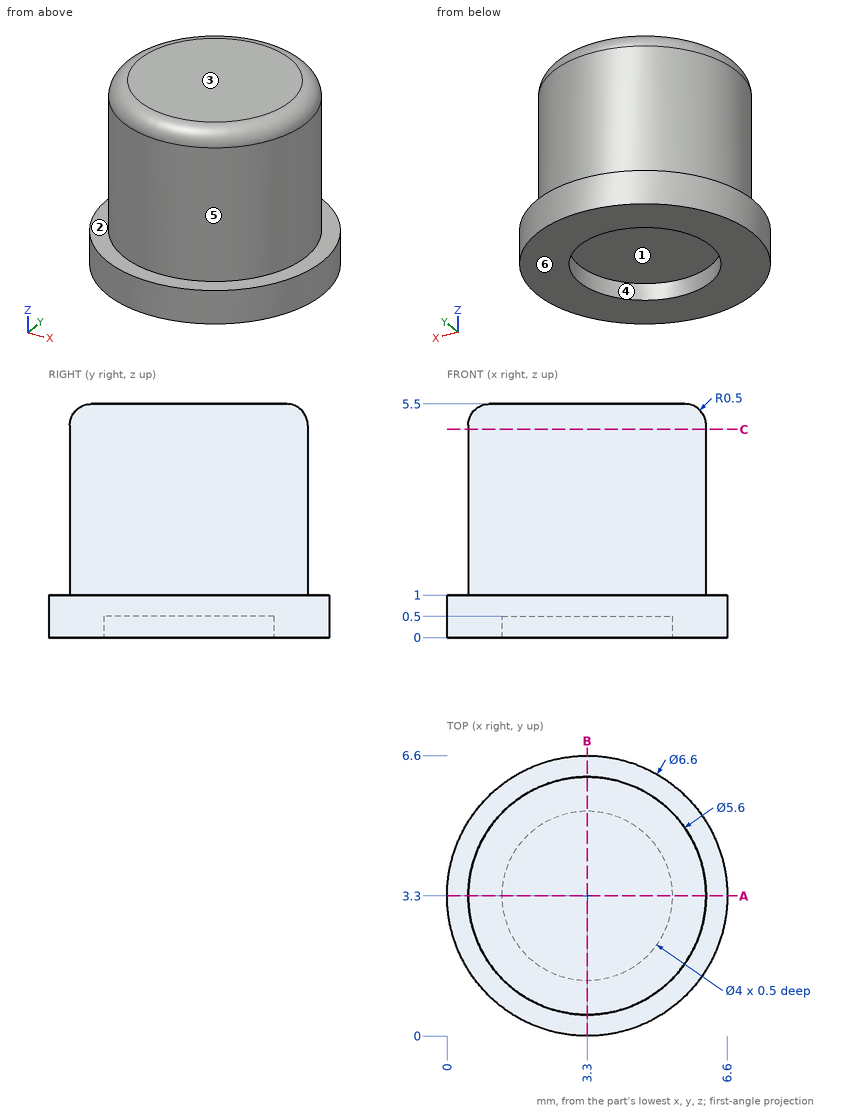
Check sheet for the drawn part. Datum: minimum x, y, z corner. Units: mm. A direction names the side the tool comes from. Round coordinates to 2 decimals unless told otherwise and drop trailing zeros. Loops run counter-clockwise (first coordinate to the right, second up) from the corner with the lowest first, then second, coordinate; pieces in that order, holes last. Notation, with made-up numbers: M 85,36.25 L 144,36.25 A27 ccw 144,75.25 Z; hole C -17.75,-39.75 d1. An arc over 180 degrees is marked long. Write each question's results on one line, items separated by ' | '.
1) Gauge pin test, flat ends, axial feed: P1, Ø2, axis at y = 2, z = 3, coming from the +X side; P2, Ø1, axis at x = 3.5, z = 4.5, coming from the -Y side; P3, Ø1, axis at x = 6, z = 4.5, coming from the +Y side. Record the tip position at first contact, or that the pin passes through.
Checks:
P1: stops at x = 6.08 | P2: stops at y = 0.5 | P3: stops at y = 5.03
2) Section check C-C on z = 4.9. Record the boundary of the cut face in (x, y), then the cut area to 3 significant figures.
Checks:
outline: C 3.3,3.3 d5.6 | area: 24.6 mm2
3) Section check A-A on y = 3.3. Record the boundary of the cut face in (x, z), then the cut area to 3 significant figures.
Checks:
outline: M 0,0 L 1.3,0 L 1.3,0.5 L 5.3,0.5 L 5.3,0 L 6.6,0 L 6.6,1 L 6.1,1 L 6.1,5 A0.5 ccw 5.6,5.5 L 1,5.5 A0.5 ccw 0.5,5 L 0.5,1 L 0,1 Z | area: 29.7 mm2
4) Scan lines: L1, parallel to Y at x = 3.3, z = 0.2; L2, parallel to Z at x = 2.5, y = 2.25; L3, parallel to Y at x = 3.25, z = 2.45. Record each from-to range of solid material in increasing order. Write a range as from..to.
Checks:
L1: y = 0..1.3, 5.3..6.6 | L2: z = 0.5..5.5 | L3: y = 0.5..6.1
5) Mould release check, pull along X, two halves, no side actions. Record for the marked faces 4, 5 and 6: released by +X, released by -X, zero draft, split by the parting line, or undercut.
Checks:
face 4: undercut | face 5: split by the parting line | face 6: zero draft
6) Access from +Z, -Z, +X, -X, +Y, -Y to the whole of each face (thin tool, end or side, straight path). Record for the marked faces 1, 2 and 3.
Checks:
face 1: -Z | face 2: +Z | face 3: +Z, +X, -X, +Y, -Y
